Here's how the part is built. I have some questions about the finished solid (model axes, mm). Face numbers are marked on the shaded views. A direction names the side the tool comes from. Round coordinates to 2 decimals unless told otherwise and drop trailing zeros. Loops run counter-clockwise (first coordinate to the right, second up) from the corner with the lowest first, then second, coordinate; pieces in that order, holes last. Notation, with made-up numbers: (28, 85) -> (83, 85) arc R22 cw to (83, 108) -> close; hole circle Ø10 at (-37.75, -34.75). An arc over 180 degrees is marked (long way). Use one line per item in the form item = value. Start each with the question number.
Item 1: If we section it at D-D (z = 2.5): Write out the boundary of the cut face in (x, y).
Item 2: Thinking about a two-plate mould opening in X: for the marked faces 1, 2, 3 and 4, which applies, released by +X, released by -X, zero draft, split by the parting line, or undercut?
Item 3: If we section it at B-B (z = 12.85): Write out the boundary of the cut face in (x, y).
Item 4: I'm going to push flat-ended pins straight in: pin 1 Ø12 at (x, y) = (-11.5, 14) entering from +Z; pin 2 Ø12 at (y, z) = (3.5, -5) entering from +X; pin 3 Ø3.5 at (x, y) = (11.95, 17.3) entering from +Z; pin 4 Ø5.5 at (x, y) = (-11.95, 17.3) entering from -Z. Where does each tip first touch, or does it pass through?
Item 5: If we section it at C-C (x = 11.95): Write out the boundary of the cut face in (y, z).
Item 6: If we section it at A-A (y = 17.3): Write out the boundary of the cut face in (x, z), then the cut area to 3 significant figures.
Item 7: For the marked faces 5, 6 and 7, which set-ups out of +Z, -Z, +X, -X, +Y, -Y let a thin tool reach every point of the face, with its end or its side?
Item 8: If I drill on L1, parallel to Y at x = -11.95, z = 8.35; L2, parallel to X at y = 1.45, z = -5.7; L3, parallel to Z at x = -6.5, y = 11.5, over which ranges is the centre line in solid material (lowest first)? Write a range as [from, to].
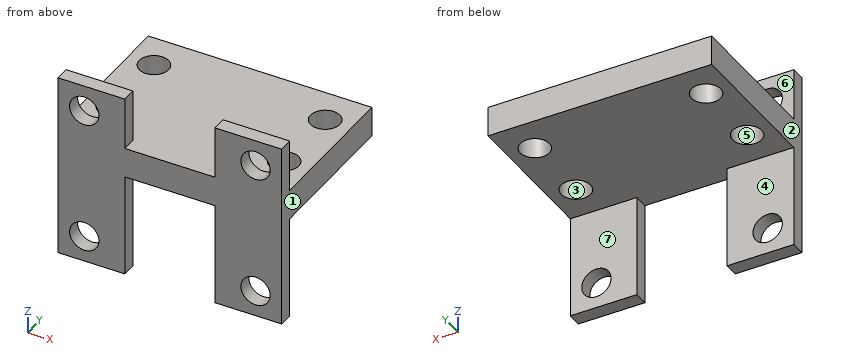
```python
from build123d import *

# Parameters (mm, degrees)
SKETCH1_R               = 2.05
BOSS_EXTRUDE1_DEPTH     = 2
BOSS_EXTRUDE2_START     = 2
BOSS_EXTRUDE2_OUTLINE_W = 31.2
BOSS_EXTRUDE2_OUTLINE_H = 4.2
BOSS_EXTRUDE2_DEPTH     = 20.4
SKETCH2_R               = 2.05
CUT_EXTRUDE1_DEPTH      = 31.838976961


# Read off the part's stored shape, not the designer's step: Boss-Extrude2
with BuildPart() as part:
    # Sketch1 → Boss-Extrude1 (new body)
    with BuildSketch(Plane(origin=(0, 0, 0), x_dir=(1, 0, 0), z_dir=(0, 1, 0))):
        Polygon((-6.3, -5), (-6.3, 9.35), (-15.6, 9.35), (-15.6, -16.5), (-6.3, -16.5), (-6.3, -9.2), (6.3, -9.2), (6.3, -16.5), (15.6, -16.5), (15.6, 9.35), (6.3, 9.35), (6.3, -5), align=None)
        with Locations(Location((11.95, -12.85, 0), (0, 0, 270))):
            Circle(SKETCH1_R, mode=Mode.SUBTRACT)
        with Locations(Location((-11.95, -12.85, 0), (0, 0, 270))):
            Circle(SKETCH1_R, mode=Mode.SUBTRACT)
        with Locations(Location((11.95, 5.7, 0), (0, 0, 270))):
            Circle(SKETCH1_R, mode=Mode.SUBTRACT)
        with Locations(Location((-11.95, 5.7, 0), (0, 0, 270))):
            Circle(SKETCH1_R, mode=Mode.SUBTRACT)
    extrude(amount=BOSS_EXTRUDE1_DEPTH)

    # Boss-Extrude2 outline → Boss-Extrude2 (add)
    with BuildSketch(Plane(origin=(0, 0, 0), x_dir=(1, 0, 0), z_dir=(0, 1, 0)).offset(BOSS_EXTRUDE2_START)):
        with Locations((0, -7.1)):
            Rectangle(BOSS_EXTRUDE2_OUTLINE_W, BOSS_EXTRUDE2_OUTLINE_H)
    extrude(amount=BOSS_EXTRUDE2_DEPTH)

    # Sketch2 → Cut-Extrude1 (cut, through all)
    with BuildSketch(Plane(origin=(0, 0, 5), x_dir=(-1, 0, 0), z_dir=(0, 0, -1))):
        with Locations((-11.95, 7.1)):
            Circle(SKETCH2_R)
        with Locations((-11.95, 17.3)):
            Circle(SKETCH2_R)
        with Locations((11.95, 7.1)):
            Circle(SKETCH2_R)
        with Locations((11.95, 17.3)):
            Circle(SKETCH2_R)
    extrude(amount=-CUT_EXTRUDE1_DEPTH, mode=Mode.SUBTRACT)


solid = part.part
```
Values found:
q1.outline = (-15.6, 0) -> (-6.3, 0) -> (-6.3, 2) -> (-15.6, 2) -> close; (6.3, 0) -> (15.6, 0) -> (15.6, 2) -> (6.3, 2) -> close
q2.face_1 = released by +X
q2.face_2 = released by -X
q2.face_3 = undercut
q2.face_4 = zero draft
q3.outline = (-15.6, 0) -> (-14, 0) -> (-14, 2) -> (-15.6, 2) -> close; (-9.9, 0) -> (-6.3, 0) -> (-6.3, 2) -> (-9.9, 2) -> close; (6.3, 0) -> (9.9, 0) -> (9.9, 2) -> (6.3, 2) -> close; (14, 0) -> (15.6, 0) -> (15.6, 2) -> (14, 2) -> close
q4.pin_1 = 9.2
q4.pin_2 = 15.6
q4.pin_3 = through
q4.pin_4 = 5
q5.outline = (0, -9.35) -> (2, -9.35) -> (2, -7.75) -> (0, -7.75) -> close; (0, -3.65) -> (2, -3.65) -> (2, 5) -> (5.05, 5) -> (5.05, 9.2) -> (2, 9.2) -> (2, 10.8) -> (0, 10.8) -> close; (0, 14.9) -> (2, 14.9) -> (2, 16.5) -> (0, 16.5) -> close; (9.15, 5) -> (15.25, 5) -> (15.25, 9.2) -> (9.15, 9.2) -> close; (19.35, 5) -> (22.4, 5) -> (22.4, 9.2) -> (19.35, 9.2) -> close
q6.outline = (-15.6, 5) -> (-14, 5) -> (-14, 9.2) -> (-15.6, 9.2) -> close; (-9.9, 5) -> (9.9, 5) -> (9.9, 9.2) -> (-9.9, 9.2) -> close; (14, 5) -> (15.6, 5) -> (15.6, 9.2) -> (14, 9.2) -> close
q6.area = 96.6 mm2
q7.face_5 = +Z, -Z
q7.face_6 = +Z, +X, -X, +Y
q7.face_7 = -Z, +X, -X, +Y
q8.L1 = [0, 5.05], [9.15, 15.25], [19.35, 22.4]
q8.L2 = [-15.6, -14], [-9.9, -6.3], [6.3, 9.9], [14, 15.6]
q8.L3 = [5, 9.2]
